Autodesk Inventor part; units mm, degrees
ref_plane "YZ Plane" through (0, 0, 0) normal (1, 0, 0) x (0, 1, 0)
ref_plane "XZ Plane" through (0, 0, 0) normal (0, 1, 0) x (-1, 0, 0)
ref_plane "XY Plane" through (0, 0, 0) normal (0, 0, 1) x (1, 0, 0)
sketch "スケッチ1" plane through (0, 0, 0) normal (0, 1, 0) x (-1, 0, 0)
  line L0 (0, 0) -> (30, 0)
  line L1 (30, 0) -> (30, -15)
  line L2 (30, -15) -> (0, -15)
  line L3 (0, -15) -> (0, 0)
  dimension "d0" = 30
  dimension "d1" = 15
extrude "押し出し1" add sketch "スケッチ1" along normal blind 300
sketch "スケッチ2" plane through (-30, 0, 0) normal (0, 0, 1) x (1, 0, 0)
  circle A0 centre (15, 45) radius 5
  line L0 (0, 0) -> (30, 0)
  line L1 (30, 0) -> (30, 300)
  dimension "d4" = 10
  dimension "d5" = 45
  dimension "d6" = 15
extrude "押し出し2" cut sketch "スケッチ2" against normal blind 300
sketch "スケッチ3" plane through (0, 0, 0) normal (0, -1, 0) x (1, 0, 0)
  line L0 (-30, 0) -> (0, 0)
  line L1 (0, 0) -> (-30, 0)
  line L2 (-30, 0) -> (-30, -15)
  line L3 (-30, -15) -> (0, -15)
  line L4 (0, -15) -> (0, 0)
  dimension "d9" = 30
  dimension "d10" = 15
extrude "押し出し3" cut sketch "スケッチ3" against normal blind 10
sketch "スケッチ5" plane through (0, 300, 0) normal (0, 1, 0) x (1, 0, 0)
  line L0 (0, 0) -> (0, 15)
  line L1 (0, 15) -> (-30, 15)
  line L2 (0, 0) -> (-30, 0)
  line L3 (-30, 0) -> (-30, 15)
  line L4 (-30, 15) -> (0, 15)
  line L5 (0, 15) -> (0, 0)
extrude "押し出し4" add sketch "スケッチ5" along normal blind 10
sketch "スケッチ6" plane through (0, 10, 0) normal (0, -1, 0) x (1, 0, 0)
  line L0 (0, 0) -> (-30, 0)
  line L1 (-30, 0) -> (-30, -15)
  line L2 (-30, -15) -> (0, -15)
  line L3 (0, -15) -> (0, 0)
extrude "押し出し5" add sketch "スケッチ6" along normal blind 60
sketch "スケッチ7" plane through (0, -50, 0) normal (0, -1, 0) x (1, 0, 0)
  line L0 (0, 0) -> (0, -15)
  line L1 (0, -15) -> (-30, -15)
  line L2 (0, 0) -> (-30, 0)
  line L3 (-30, 0) -> (-30, -15)
  line L4 (-30, -15) -> (0, -15)
  line L5 (0, -15) -> (0, 0)
extrude "押し出し6" cut sketch "スケッチ7" against normal blind 5
sketch "スケッチ8" plane through (-30, 310, 0) normal (0, 0, 1) x (1, 0, 0)
  circle A0 centre (15, -265) radius 6
  line L0 (0, -355) -> (30, -355)
  line L1 (0, -355) -> (0, 0)
  circle A1 centre (15, -265) radius 5
  point P0 (30, -310)
  dimension "d19" = 12
  dimension "d20" = 90
  dimension "d21" = 15
  dimension "d22" = 10
extrude "押し出し7" cut sketch "スケッチ8" against normal blind 15
sketch "スケッチ9" plane through (0, 310, 0) normal (0, 1, 0) x (1, 0, 0)
  line L0 (-28.5, 13.5) -> (-1.5, 13.5)
  line L1 (-1.5, 13.5) -> (-1.5, 1.5)
  line L2 (-1.5, 1.5) -> (-28.5, 1.5)
  line L3 (-28.5, 1.5) -> (-28.5, 13.5)
  line L4 (0, 15) -> (-30, 15)
  line L5 (-30, 15) -> (-30, 0)
  point P0 (0, 0)
  dimension "d25" = 27
  dimension "d26" = 12
  dimension "d27" = 1.5
  dimension "d28" = 1.5
extrude "押し出し8" cut sketch "スケッチ9" against normal blind 500
properties part number "射出_腕" material "アルミニウム 6061"
Verification items for the finished model (mm, model axes). A direction names the side the tool comes from. Give positions to 0.01 mm unless a question says otherwise; leave off trailing zeros. Write each loop counter-clockwise with the first axis right and the second up, starting at its lowest first coordinate (ties: lowest second). Pieces come first, ordered by that corner, then holes. Notation, with made-up numbers: M 63,-31 L 115,-31 A9 ccw 115,-20 Z; hole C 36.5,-14 d10. An arc over 180 degrees is marked long. Use CSV: the item, a comma, the result in double quotes.
1) Cross-section at B-B (z = -9.5). Enter the section's corners in (x, y).
Final values:
outline,"M -30,-45 L -28.5,-45 L -28.5,310 L -30,310 Z; M -1.5,-45 L 0,-45 L 0,310 L -1.5,310 Z"
2) Cross-section at D-D (y = 267). Enter the section's corners in (x, z), plus the area to 3 significant figures.
Final values:
outline,"M -30,-15 L 0,-15 L 0,0 L -30,0 Z; hole M -28.5,-13.5 L -1.5,-13.5 L -1.5,-1.5 L -28.5,-1.5 Z"
area,"126 mm²"
3) Material ranges on line 1 along Z through (x, y) = (-27, 211); line 2 along X through (y, z) = (229, -9.75); line 3 along Y through (x, z) = (-15, -0.7), recorded low to high.
Final values:
line 1,"-15 to -13.5, -1.5 to 0"
line 2,"-30 to -28.5, -1.5 to 0"
line 3,"-45 to 39, 51 to 310"
4) Cross-section at C-C (x = -15). Enter the section's corners in (y, z), plus the area to 3 significant figures.
Final values:
outline,"M -45,-15 L 39,-15 L 39,-13.5 L -45,-13.5 Z; M -45,-1.5 L 39,-1.5 L 39,0 L -45,0 Z; M 51,-15 L 310,-15 L 310,-13.5 L 51,-13.5 Z; M 51,-1.5 L 310,-1.5 L 310,0 L 51,0 Z"
area,"1,030 mm²"
5) Cross-section at A-A (y = 45). Enter the section's corners in (x, z).
Final values:
outline,"M -30,-15 L -21,-15 L -21,-13.5 L -28.5,-13.5 L -28.5,-1.5 L -21,-1.5 L -21,0 L -30,0 Z; M -9,-15 L 0,-15 L 0,0 L -9,0 L -9,-1.5 L -1.5,-1.5 L -1.5,-13.5 L -9,-13.5 Z"
6) Access from +Z, -Z, +X, -X, +Y, -Y to the whole of each face (thin tool, end or side, straight path). Record for faces 5 (the face through (-1.5, 135, -8)), 6 (the face through (-30, 135, -7)).
Final values:
face 5,"+Y, -Y"
face 6,"+Z, -Z, -X, +Y, -Y"
7) Release check for a two-part mould opening along X. For faces 1 (the face through (-9.46, 42.7, -0.74)), 2 (the face through (0, 135, -8)), 3 (the face through (-15, 135, -1.5)), 4 (the face through (-15, 135, 0)) record: released by +X, released by -X, zero draft, split by the parting line, or undercut.
Final values:
face 1,"undercut"
face 2,"released by +X"
face 3,"undercut"
face 4,"zero draft"
